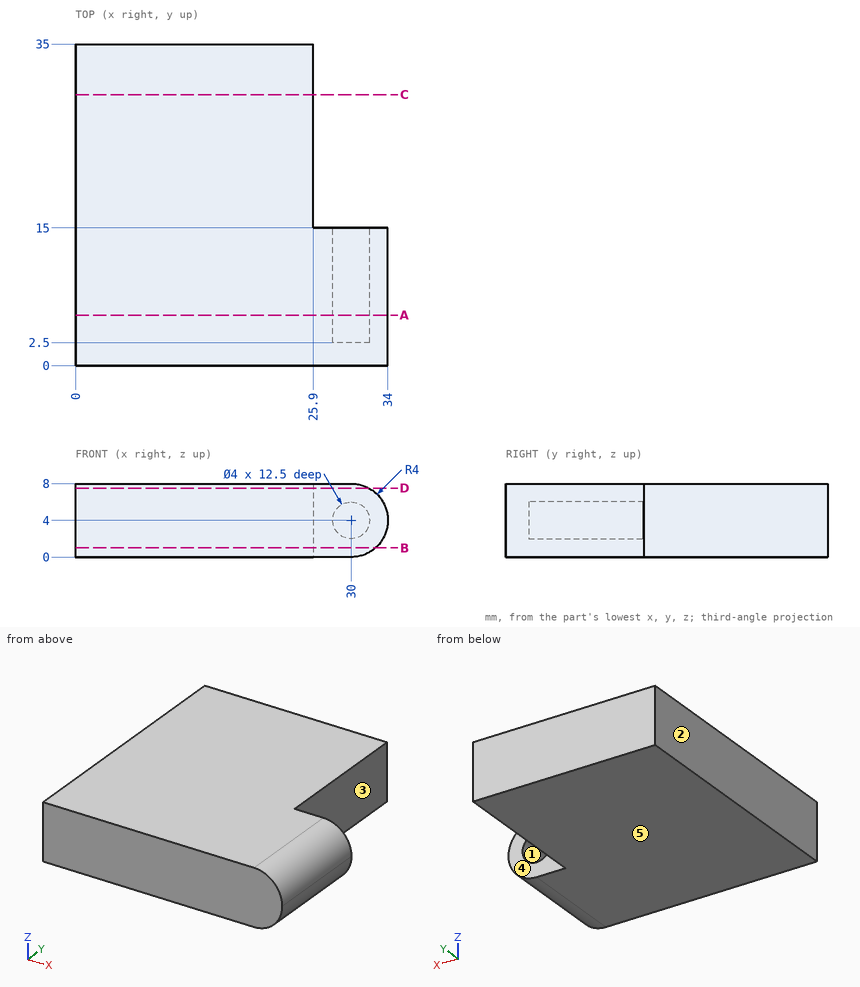
Can you work these out from the drawing? Everything is in mm from the part's minimum corner. A direction names the side the tool comes from. Give positions to 0.01 mm unless a question says otherwise; leave off trailing zeros. Write each loop counter-clockwise with the first axis right and the second up, starting at its lowest first coordinate (ties: lowest second). Pieces come first, ordered by that corner, then holes. Notation, with made-up numbers: M 37.5,25.5 L 95.5,25.5 A17 ccw 95.5,33.5 Z; hole C 0.5,6.25 d2. An arc over 180 degrees is marked long. Answer in a Markdown table with one row per item. Add a question column.
Item 1: On a 3-axis mill with a long thin cutter (end or side, diameter ignored), from which of +Z, -Z, +X, -X, +Y, -Y can I reach the whole of each face in a straight line? I mean the marked faces 4 and 5. Say none if no direction works.
Item 2: Imagine slicing it at D-D, the plane z = 7.5. Write out the boundary of the cut face in (x, y), plus the area to 3 significant figures.
Item 3: Please list where these lines run through material, in increasing order: L1, parallel to X at y = 12, z = 4; L2, parallel to Y at x = 30.5, z = 3.25; L3, parallel to Y at x = 31.5, z = 6.25.
Item 4: Imagine slicing it at A-A, the plane y = 5.5. Write out the boundary of the cut face in (x, z).
Item 5: For pin 1 Ø2.5 at (x, z) = (30, 4) entering from +Y, with a flat end and sliding along its axis, tell me the tip position at first contact or that it passes through.
Item 6: We'd pull the mould along X, two halves only. Please class the marked faces 1, 2 and 3: released by +X, released by -X, zero draft, split by the parting line, or undercut.
Item 7: Imagine slicing it at C-C, the plane y = 29.5. Write out the boundary of the cut face in (x, z).
Item 8: Imagine slicing it at B-B, the plane z = 1. Write out the boundary of the cut face in (x, y).
Evaluation:
| question | item | result |
|---|---|---|
| 1 | face 4 | +Z, -Z, +X, +Y |
| 1 | face 5 | -Z, +X, -X, +Y, -Y |
| 2 | outline | M 0,0 L 31.94,0 L 31.94,15 L 25.9,15 L 25.9,35 L 0,35 Z |
| 2 | area | 997 mm² |
| 3 | L1 | x = 0 to 28, 32 to 34 |
| 3 | L2 | y = 0 to 2.5 |
| 3 | L3 | y = 0 to 15 |
| 4 | outline | M 0,0 L 30,0 A4 ccw 30,8 L 0,8 Z; hole C 30,4 d4 |
| 5 | pin 1 | stops at y = 2.5 |
| 6 | face 1 | undercut |
| 6 | face 2 | released by -X |
| 6 | face 3 | released by +X |
| 7 | outline | M 0,0 L 25.9,0 L 25.9,8 L 0,8 Z |
| 8 | outline | M 0,0 L 32.65,0 L 32.65,15 L 25.9,15 L 25.9,35 L 0,35 Z |
